Model file for the job. Use its own axes, mm. A direction names the side the tool comes from. Give positions to 0.01 mm unless a question says otherwise; leave off trailing zeros. Write each loop counter-clockwise with the first axis right and the second up, starting at its lowest first coordinate (ties: lowest second). Pieces come first, ordered by that corner, then holes.
Autodesk Inventor part; units mm, degrees
ref_plane "YZ Plane" through (0, 0, 0) normal (1, 0, 0) x (0, 1, 0)
ref_plane "XZ Plane" through (0, 0, 0) normal (0, 1, 0) x (-1, 0, 0)
ref_plane "XY Plane" through (0, 0, 0) normal (0, 0, 1) x (1, 0, 0)
sketch "スケッチ1" plane through (0, 0, 0) normal (1, 0, 0) x (0, 1, 0)
  line L0 (7, 15) -> (-7, 15)
  line L1 (-7, 15) -> (-7, -15)
  line L2 (-7, -15) -> (7, -15)
  line L3 (7, -15) -> (7, 15)
  circle A0 centre (0, 10.05) radius 1.5
  circle A1 centre (0, -11.55) radius 1.5
  point P0 (0, 0)
  dimension "d0" = 14
  dimension "d1" = 30
  dimension "d2" = 7
  dimension "d3" = 15
  dimension "d4" = 3
  dimension "d5" = 3
  dimension "d6" = 3.45
  dimension "d7" = 3.45
extrude "押し出し1" add sketch "スケッチ1" along normal blind 1.6
sketch "スケッチ2" plane through (1.6, 0, 0) normal (1, 0, 0) x (0, 0, -1)
  line L0 (-2, 2.5) -> (2, 2.5)
  line L1 (2, 2.5) -> (2, -2.5)
  line L2 (2, -2.5) -> (-2, -2.5)
  line L3 (-2, -2.5) -> (-2, 2.5)
  point P0 (0, 0)
  dimension "d10" = 4
  dimension "d11" = 5
  dimension "d12" = 2.5
  dimension "d13" = 2
extrude "押し出し2" add sketch "スケッチ2" along normal blind 1.6
sketch "スケッチ3" plane through (0, 0, 0) normal (-1, 0, 0) x (0, 0, 1)
  line L0 (6.25, -5.725) -> (-6.25, -5.725)
  line L1 (-6.25, -5.725) -> (-6.25, 5.725)
  line L2 (-6.25, 5.725) -> (6.25, 5.725)
  line L3 (6.25, 5.725) -> (6.25, -5.725)
  line L4 (-15, -7) -> (-15, 7)
  line L5 (15, 7) -> (15, -7)
  point P0 (0, 0)
  dimension "d16" = 12.5
  dimension "d17" = 8.75
  dimension "d18" = 8.75
  dimension "d19" = 11.45
  dimension "d20" = 5.725
  dimension "d21" = 5.725
extrude "押し出し3" add sketch "スケッチ3" along normal blind 6
chamfer "面取り1" distance 4 angle 45 1 edges at (-6, -5.725, 0)
properties part number "encoder"
1. Slice it at A-A, the plane z = -11.55. Write the cut outline in (x, y), and give its area (3 significant figures).
Calculated:
outline: (0, -7) - (1.6, -7) - (1.6, -1.5) - (0, -1.5) - close; (0, 1.5) - (1.6, 1.5) - (1.6, 7) - (0, 7) - close
area: 17.6 mm2
2. Pull direction Z, two halves, no side cores. Call faces 5 (the flat face through (-3, 0, 6.25)), 6 (the cylindrical face through (0.789, -0.325, -10.086)), 7 (the flat face through (1, 7, 0)), 8 (the cylindrical face through (0.789, -0.325, 11.514)): +Z half, -Z half, draft (parallel to the pull), parting line (faces both ways), or undercut.
Calculated:
face 5: +Z half
face 6: undercut
face 7: draft
face 8: undercut
3. Slice it at B-B, the plane y = 0. Write the cut outline in (x, z).
Calculated:
outline: (-6, -6.25) - (0, -6.25) - (0, -10.05) - (1.6, -10.05) - (1.6, -2) - (3.2, -2) - (3.2, 2) - (1.6, 2) - (1.6, 8.55) - (0, 8.55) - (0, 6.25) - (-6, 6.25) - close; (0, -15) - (1.6, -15) - (1.6, -13.05) - (0, -13.05) - close; (0, 11.55) - (1.6, 11.55) - (1.6, 15) - (0, 15) - close
4. Which spindle directions (+Z, -Z, +X, -X, +Y, -Y) get a long thin tool onto all of the face, cutting with end or side? Do faces 1 (the flat face through (2, 0, -2)), 2 (the flat face through (-3, 5.725, 0)), 3 (the flat face through (2, 2.5, 0)), 4 (the flat face through (-3, 0, -6.25)). Say none if no direction does.
Calculated:
face 1: -Z, +X, +Y, -Y
face 2: +Z, -Z, -X, +Y
face 3: +Z, -Z, +X, +Y
face 4: -Z, -X, +Y, -Y
5. Pin check, flat tips, straight feed: P1, Ø0.8, axis at x = 2.5, y = -1, coming from the -Z side; P2, Ø1.6, axis at x = -0.5, z = 0.5, coming from the -Y side; P3, Ø1.3, axis at x = 2.5, z = 1, coming from the +Y side; P4, Ø0.8, axis at x = 2.5, z = 0.5, coming from the -Y side. Stop position of each tip, or through.
Calculated:
P1: stops at z = -2
P2: stops at y = -7
P3: stops at y = 2.5
P4: stops at y = -2.5
6. Slice it at D-D, the plane z = 4.75. Write the cut outline in (x, y) (3 decimals), and give its area (3 significant figures).
Calculated:
outline: (-6, -1.725) - (-2, -5.725) - (0, -5.725) - (0, -7) - (1.6, -7) - (1.6, 7) - (0, 7) - (0, 5.725) - (-6, 5.725) - close
area: 83.1 mm2
7. Probe probe 1 along Z at (x, y) = (1.35, 0); probe 2 along X at (y, z) = (-6.25, -6.25); probe 3 along X at (y, z) = (-1.25, -6). List the from-to ranges inside material, lowest first.
Calculated:
probe 1: z = -15 to -13.05, -10.05 to 8.55, 11.55 to 15
probe 2: x = 0 to 1.6
probe 3: x = -6 to 1.6
8. Slice it at C-C, the plane y = 2. Write the cut outline in (x, z).
Calculated:
outline: (-6, -6.25) - (0, -6.25) - (0, -15) - (1.6, -15) - (1.6, -2) - (3.2, -2) - (3.2, 2) - (1.6, 2) - (1.6, 15) - (0, 15) - (0, 6.25) - (-6, 6.25) - close
